Source: CAD feature listing. Evaluate the final solid. Frame: model axes, mm. Give positions to 0.01 mm unless a question says otherwise; leave off trailing zeros. Write each loop counter-clockwise with the first axis right and the second up, starting at its lowest first coordinate (ties: lowest second). Pieces come first, ordered by that corner, then holes. Notation, with made-up numbers: (78.25, -13.75) -> (104.25, -13.75) arc R18 ccw to (104.25, -7.75) -> close; hole circle Ø2 at (53, 65). An arc over 180 degrees is marked (long way). Write item = value, one per line.
from build123d import *

# Parameters (mm, degrees)
SKETCH1_W           = 363.22
SKETCH1_H           = 152.4
SKETCH1_R           = 3.6703
SKETCH1_R_2         = 2.921
BOSS_EXTRUDE1_DEPTH = 6.35
SKETCH2_W           = 6.35
SKETCH2_H           = 6.35
SKETCH2_H_2         = 19.05000003
SKETCH2_H_3         = 19.05
CUT_EXTRUDE1_DEPTH  = 7.35
SKETCH5_R           = 1.5
CUT_EXTRUDE2_DEPTH  = 7.35
SKETCH7_R           = 1.651
CUT_EXTRUDE3_DEPTH  = 7.35
SKETCH8_R           = 1.75
CUT_EXTRUDE4_DEPTH  = 7.35
SKETCH9_R           = 1.25
CUT_EXTRUDE5_DEPTH  = 7.35
SKETCH10_R          = 1.25
CUT_EXTRUDE6_DEPTH  = 7.35


with BuildPart() as part:
    # Sketch1 → Boss-Extrude1 (new body)
    with BuildSketch(Plane(origin=(0, 0, 0), x_dir=(1, 0, 0), z_dir=(0, 1, 0))):
        with Locations((181.61, 76.2)):
            Rectangle(SKETCH1_W, SKETCH1_H)
        with Locations((25.4, 63.5)):
            Circle(SKETCH1_R, mode=Mode.SUBTRACT)
        with Locations((25.4, 88.9)):
            Circle(SKETCH1_R, mode=Mode.SUBTRACT)
        with Locations((353.06, 60.325)):
            Circle(SKETCH1_R_2, mode=Mode.SUBTRACT)
        with Locations((353.06, 92.075)):
            Circle(SKETCH1_R_2, mode=Mode.SUBTRACT)
    extrude(amount=BOSS_EXTRUDE1_DEPTH)

    # Sketch2 → Cut-Extrude1 (cut, through all)
    with BuildSketch(Plane(origin=(0, 6.35, 0), x_dir=(1, 0, 0), z_dir=(0, 1, 0))):
        with Locations((25.4, 104.775)):
            Rectangle(SKETCH2_W, SKETCH2_H)
        with Locations((25.4, 47.625)):
            Rectangle(SKETCH2_W, SKETCH2_H)
        with Locations((32.2453, 76.2)):
            Rectangle(SKETCH2_W, SKETCH2_H_2)
        with Locations((18.5547, 76.199999985)):
            Rectangle(SKETCH2_W, SKETCH2_H_3)
        with Locations((114.7953, 76.2)):
            Rectangle(SKETCH2_W, SKETCH2_H_2)
    extrude(amount=-CUT_EXTRUDE1_DEPTH, mode=Mode.SUBTRACT)

    # Sketch5 → Cut-Extrude2 (cut, through all)
    with BuildSketch(Plane(origin=(0, 6.35, 0), x_dir=(1, 0, 0), z_dir=(0, 1, 0))):
        with Locations((79.4639, 6.096)):
            Circle(SKETCH5_R)
    extrude(amount=-CUT_EXTRUDE2_DEPTH, mode=Mode.SUBTRACT)

    # Sketch7 → Cut-Extrude3 (cut, through all)
    with BuildSketch(Plane(origin=(0, 6.35, 0), x_dir=(1, 0, 0), z_dir=(0, 1, 0))):
        with Locations((138.807883042, 134.62)):
            Circle(SKETCH7_R)
        with Locations((255.647883042, 134.62)):
            Circle(SKETCH7_R)
        with Locations((255.647883042, 17.78)):
            Circle(SKETCH7_R)
        with Locations((138.807883042, 17.78)):
            Circle(SKETCH7_R)
    extrude(amount=-CUT_EXTRUDE3_DEPTH, mode=Mode.SUBTRACT)

    # Sketch8 → Cut-Extrude4 (cut, through all)
    with BuildSketch(Plane(origin=(0, 6.35, 0), x_dir=(1, 0, 0), z_dir=(0, 1, 0))):
        with Locations((321.047883042, 96.2)):
            Circle(SKETCH8_R)
        with Locations((281.047883042, 56.2)):
            Circle(SKETCH8_R)
    extrude(amount=-CUT_EXTRUDE4_DEPTH, mode=Mode.SUBTRACT)

    # Sketch9 → Cut-Extrude5 (cut, through all)
    with BuildSketch(Plane(origin=(0, 6.35, 0), x_dir=(1, 0, 0), z_dir=(0, 1, 0))):
        with Locations((18.5547, 92.074999985)):
            Circle(SKETCH9_R)
        with Locations((32.2453, 92.075000015)):
            Circle(SKETCH9_R)
        with Locations((32.2453, 60.324999985)):
            Circle(SKETCH9_R)
        with Locations((18.5547, 60.324999985)):
            Circle(SKETCH9_R)
        with Locations((114.7953, 92.075000015)):
            Circle(SKETCH9_R)
        with Locations((114.7953, 60.324999985)):
            Circle(SKETCH9_R)
    extrude(amount=-CUT_EXTRUDE5_DEPTH, mode=Mode.SUBTRACT)

    # Sketch10 → Cut-Extrude6 (cut, through all)
    with BuildSketch(Plane(origin=(0, 6.35, 0), x_dir=(1, 0, 0), z_dir=(0, 1, 0))):
        with Locations((60.8203, 87.2)):
            Circle(SKETCH10_R)
        with Locations((72.8203, 87.2)):
            Circle(SKETCH10_R)
        with Locations((72.8203, 65.2)):
            Circle(SKETCH10_R)
        with Locations((60.8203, 65.2)):
            Circle(SKETCH10_R)
    extrude(amount=-CUT_EXTRUDE6_DEPTH, mode=Mode.SUBTRACT)


solid = part.part
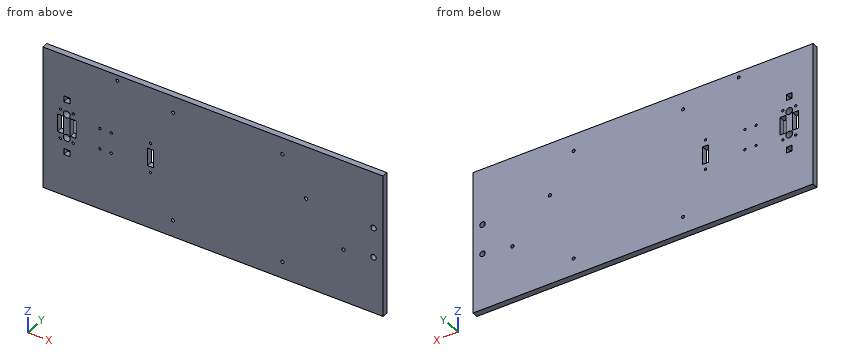
1) Cut plane A-A (z = -75.5). Return the cut outline in (x, y), then the cut area to 3 significant figures.
Computed:
outline = (0, 0) -> (15.38, 0) -> (15.38, 6.35) -> (0, 6.35) -> close; (21.73, 0) -> (29.07, 0) -> (29.07, 6.35) -> (21.73, 6.35) -> close; (35.42, 0) -> (111.62, 0) -> (111.62, 6.35) -> (35.42, 6.35) -> close; (117.97, 0) -> (363.22, 0) -> (363.22, 6.35) -> (117.97, 6.35) -> close
area = 2,190 mm²
2) Material intervals for L1, parallel to Z at x = 25.4, y = 3.5; L2, parallel to X at y = 6.25, z = -86.5; L3, parallel to X at y = 2.25, z = -88.9, sorted ascending.
Computed:
L1 = -152.4 to -107.95, -101.6 to -92.57, -85.23 to -67.17, -59.83 to -50.8, -44.45 to 0
L2 = 0 to 22.62, 28.18 to 59.78, 61.86 to 71.78, 73.86 to 363.22
L3 = 0 to 21.73, 29.07 to 363.22
3) Cut plane B-B (x = 25.4). Return the cut outline in (y, z).
Computed:
outline = (0, -152.4) -> (6.35, -152.4) -> (6.35, -107.95) -> (0, -107.95) -> close; (0, -101.6) -> (6.35, -101.6) -> (6.35, -92.57) -> (0, -92.57) -> close; (0, -85.23) -> (6.35, -85.23) -> (6.35, -67.17) -> (0, -67.17) -> close; (0, -59.83) -> (6.35, -59.83) -> (6.35, -50.8) -> (0, -50.8) -> close; (0, -44.45) -> (6.35, -44.45) -> (6.35, 0) -> (0, 0) -> close
